Geometry check sheet. Reference: drawing and pictorial views, mm from the part's lowest x, y, z. A direction names the side the tool comes from. Give positions to 0.01 mm unless a question says otherwise; leave off trailing zeros. Write each loop counter-clockwise with the first axis right and the second up, starting at its lowest first coordinate (ties: lowest second). Pieces come first, ordered by that corner, then holes. Notation, with made-up numbers: M 19,42 L 71,42 A27 cw 71,73 Z; hole C -8.75,29.25 d9. An arc over 180 degrees is marked long. Write item = value, one per line. Start each with the question number.
1) Cross-section at C-C, the plane x = 10. Record the cut outline in (y, z), plus the area to 3 significant figures.
2) Scan lines: line 1 along X through (y, z) = (2, 2.75) (3 decimals); line 2 along X through (y, z) = (7, 1.5) (3 decimals); line 3 along Z through (x, y) = (5.5, 6). Record each from-to range of solid material in increasing order. Write a range as [from, to].
3) Access from +Z, -Z, +X, -X, +Y, -Y to the whole of each face (thin tool, end or side, straight path). Record for the marked faces 1, 2 and 3.
4) Go/stop test with flat-tipped pins: pin 1 (1 mm diameter, centred on x = 22.5, z = 1.5, fed in from +Y); pin 2 (2 mm diameter, centred on y = 2.5, z = 4, fed in from -X); pin 3 (2 mm diameter, centred on x = 15.5, z = 9.5, fed in from +Y). Record where each tip stops, or that it passes through.
5) Mould release check, pull along X, two halves, no side actions. Record for the marked faces 4, 5 and 6: released by +X, released by -X, zero draft, split by the parting line, or undercut.
6) Cross-section at A-A, the plane y = 6. Record the cut outline in (x, z) (3 decimals), plus the area to 3 significant figures.
7) Cross-section at D-D, the plane x = 17.5. Record the cut outline in (y, z).
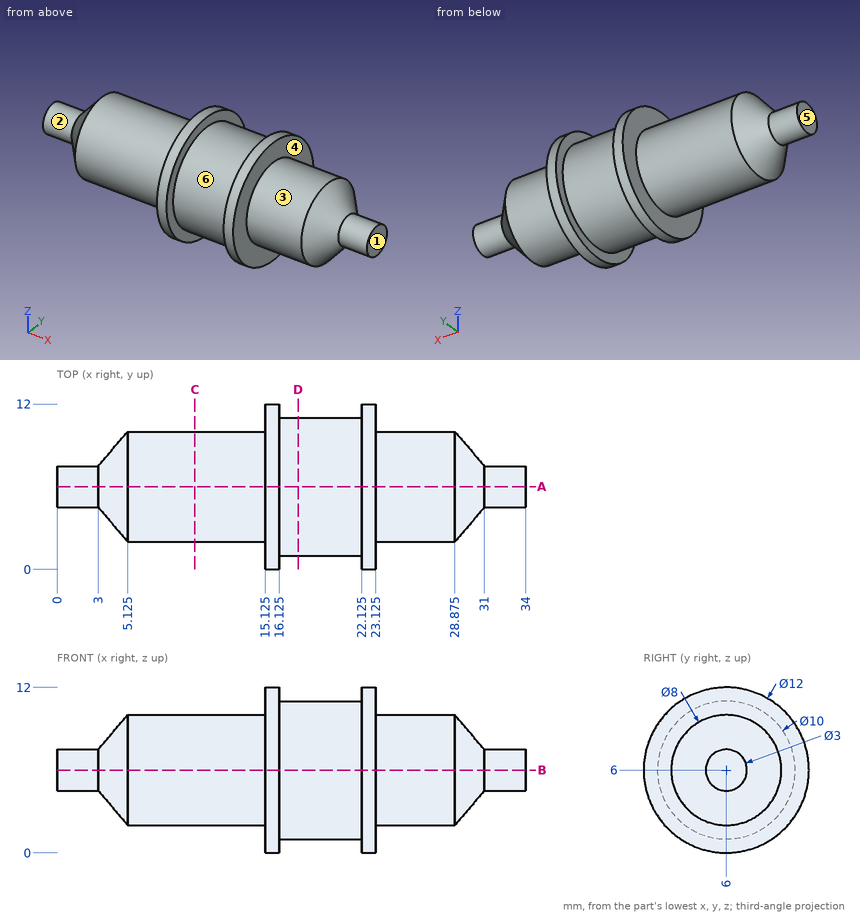
Reply:
q1.outline = C 6,6 d8
q1.area = 50.3 mm2
q2.line_1 = [15.125, 16.125], [22.125, 23.125]
q2.line_2 = [15.125, 23.125]
q2.line_3 = [2, 10]
q3.face_1 = +Z, -Z, +X, +Y, -Y
q3.face_2 = -X
q3.face_3 = +X
q4.pin_1 = 10.47
q4.pin_2 = 4.3
q4.pin_3 = 11.45
q5.face_4 = released by +X
q5.face_5 = released by -X
q5.face_6 = undercut
q6.outline = M 0,4.5 L 3,4.5 L 5.125,2 L 15.125,2 L 15.125,0 L 16.125,0 L 16.125,1 L 22.125,1 L 22.125,0 L 23.125,0 L 23.125,2 L 28.875,2 L 31,4.5 L 34,4.5 L 34,7.5 L 31,7.5 L 28.875,10 L 23.125,10 L 23.125,12 L 22.125,12 L 22.125,11 L 16.125,11 L 16.125,12 L 15.125,12 L 15.125,10 L 5.125,10 L 3,7.5 L 0,7.5 Z
q6.area = 251 mm2
q7.outline = C 6,6 d10
